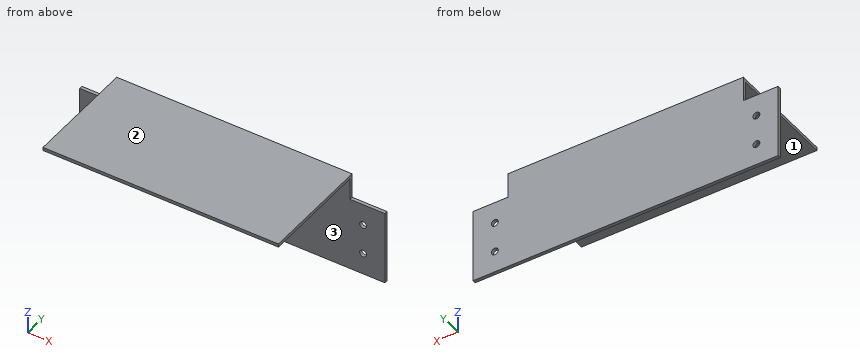
```python
from build123d import *

# Parameters (mm, degrees)
BOSS_EXTRUDE1_OUTLINE_R = 1.5875
BOSS_EXTRUDE1_DEPTH     = 1.5
SKETCH2_W               = 108
SKETCH2_H               = 1.5
BOSS_EXTRUDE2_DEPTH     = 50


# Read off the part's stored shape, not the designer's step: Boss-Extrude1
with BuildPart() as part:
    # Boss-Extrude1 outline → Boss-Extrude1 (new body)
    with BuildSketch(Plane(origin=(0, 0, 0), x_dir=(1, 0, 0), z_dir=(0, 1, 0))):
        Polygon((84.421900247, 14.871495129), (84.421900247, 26.371495129), (100.421900247, 26.371495129), (100.421900247, 60.371495129), (-39.578099753, 60.371495129), (-39.578099753, 26.371495129), (-23.578099753, 26.371495129), (-23.578099753, 14.871495129), align=None)
        with Locations((-29.578099753, 36.371495129)):
            Circle(BOSS_EXTRUDE1_OUTLINE_R, mode=Mode.SUBTRACT)
        with Locations((90.421900247, 36.371495129)):
            Circle(BOSS_EXTRUDE1_OUTLINE_R, mode=Mode.SUBTRACT)
        with Locations((-29.578099753, 50.371495129)):
            Circle(BOSS_EXTRUDE1_OUTLINE_R, mode=Mode.SUBTRACT)
        with Locations((90.421900247, 50.371495129)):
            Circle(BOSS_EXTRUDE1_OUTLINE_R, mode=Mode.SUBTRACT)
    extrude(amount=BOSS_EXTRUDE1_DEPTH)

    # Sketch2 → Boss-Extrude2 (add)
    with BuildSketch(Plane.XZ):
        with Locations((30.421900247, -15.621495129)):
            Rectangle(SKETCH2_W, SKETCH2_H)
    extrude(amount=BOSS_EXTRUDE2_DEPTH)


solid = part.part
```
Verification items for the finished model (mm, model axes). Face numbers are marked on the shaded views. Coordinates: 2 decimals unless noted, no trailing zeros. Write each loop counter-clockwise with the first axis right and the second up, starting at its lowest first coordinate (ties: lowest second). Pieces come first, ordered by that corner, then holes. Notation, with made-up numbers: (-5.5, 27) - (25.5, 27) arc R22 ccw to (25.5, 43) - close; hole circle Ø4 at (19, -20). An arc over 180 degrees is marked (long way). One line per question, with ' | ' between items. Start each with the question number.
1. Draft check along Z on the marked faces 1, 2 and 3. Enter one of: released by +Z, released by -Z, zero draft, split by the parting line, or undercut.
2. Section check A-A (z = -18). Enter the section's corners in (x, y).
3. Section check B-B (x = -18.5). Enter the section's corners in (y, z), plus the area to 3 significant figures.
4. Gauge pin test, flat ends, axial feed: P1, Ø3.5, axis at x = -29.58, z = -36.37, coming from the +Y side; P2, Ø6, axis at y = -32.5, z = -19, coming from the -X side; P3, Ø4, axis at x = 90.42, z = -36.37, coming from the -Y side; P4, Ø2, axis at x = 55, y = -35, coming from the -Z side. Record the tip position at first contact, or that the pin passes through.
5. Section check C-C (y = -23). Enter the section's corners in (x, z).
6. Material ranges on line 1 along Y through (x, z) = (75, -30); line 2 along Z through (x, y) = (9, -31), recorded low to high.
Computed values:
1) face 1: released by -Z | face 2: released by +Z | face 3: zero draft
2) outline: (-23.58, 0) - (84.42, 0) - (84.42, 1.5) - (-23.58, 1.5) - close
3) outline: (-50, -16.37) - (0, -16.37) - (0, -60.37) - (1.5, -60.37) - (1.5, -14.87) - (-50, -14.87) - close | area: 143 mm²
4) P1: y = 1.5 | P2: x = -23.58 | P3: y = 0 | P4: z = -16.37
5) outline: (-23.58, -16.37) - (84.42, -16.37) - (84.42, -14.87) - (-23.58, -14.87) - close
6) line 1: 0 to 1.5 | line 2: -16.37 to -14.87
